Build history of the part. All positions in model axes, mm. A direction names the side the tool comes from. Give positions to 0.01 mm unless a question says otherwise; leave off trailing zeros. Write each loop counter-clockwise with the first axis right and the second up, starting at its lowest first coordinate (ties: lowest second). Pieces come first, ordered by that corner, then holes. Notation, with made-up numbers: (16.5, 11) -> (57.5, 11) arc R11 cw to (57.5, 26) -> close; hole circle Ø3 at (-6, -34.5). An arc over 180 degrees is marked (long way). Put each result on its own line as item: value. Start each with the question number.
Item 1: Flat gauge pins, fed straight in: pin 1 Ø1.4 at (x, z) = (39.5, 1) entering from +Y; pin 2 Ø1 at (x, z) = (-14.5, 2.5) entering from -Y; pin 3 Ø0.8 at (y, z) = (6.5, 1) entering from +X. Where does each tip first touch, or does it go through?
Item 2: Tool access for faces 4 (the flat face through (55.75, -20, 1)), 5 (the flat face through (-17.9, 10, 1)), 6 (the flat face through (0, 26.75, 1)), 7 (the flat face through (29, -26.75, 1)), 8 (the flat face through (17.9, 9, 1)): list every direction of +Z, -Z, +X, -X, +Y, -Y with a clear straight run to the whole face (end or side of a thin tool).
Item 3: Two-plate mould, pull along Y, no slides. Class faces 1 (the cylindrical face through (-4.1, -27.144, 1.38)), 2 (the cylindrical face through (-20.03, -10.26, 0.81)), 3 (the cylindrical face through (24, -12.68, 1.38)): pulls with the +Y half, pulls with the -Y half, needs draft (parallel to the pull), parting line crosses it, or undercut.
Item 4: Drill centre lines: line 1 along X through (y, z) = (-11.25, 1.1); line 2 along X through (y, z) = (-11.25, 2.75); line 3 along Y through (x, z) = (-19.9, 1.05). Where is each one in solid material? Low to high.
Item 5: Slice it at C-C, the plane x = -35. List the corners of the cut face in (y, z), plus the area to 3 significant figures.
Item 6: Slice it at A-A, the plane z = 0.55. List the corners of the cut face in (x, y).
Item 7: Slice it at B-B, the plane y = 3. List the corners of the cut face in (x, z).
```python
from build123d import *

# Parameters (mm, degrees)
BOSS_EXTRUDE1_DEPTH                            = 2.8
CUT_EXTRUDE1_REACH                             = 4.8
SKETCH3_R                                      = 1
CSK_FOR_M2_FLAT_HEAD_MACHINE_SCREW1_AT_2_COUNT = 2
CSK_FOR_M2_FLAT_HEAD_MACHINE_SCREW1_AT_2_PITCH = 39.8


with BuildPart() as part:
    # Sketch1 → Boss-Extrude1 (new body)
    with BuildSketch(Plane.XY):
        with BuildLine():
            Line((-53.75, -26.75), (-5.291502622, -26.75))
            ThreePointArc((-5.291502622, -26.75), (-4.085457244, -27.15455193), (-3.36731985, -28.204545455))
            ThreePointArc((-3.36731985, -28.204545455), (0, -30.75), (3.36731985, -28.204545455))
            ThreePointArc((3.36731985, -28.204545455), (4.085457244, -27.15455193), (5.291502622, -26.75))
            Line((5.291502622, -26.75), (53.75, -26.75))
            ThreePointArc((53.75, -26.75), (55.164213562, -26.164213562), (55.75, -24.75))
            Line((55.75, -24.75), (55.75, -15.25))
            ThreePointArc((55.75, -15.25), (55.164213562, -13.835786438), (53.75, -13.25))
            Line((53.75, -13.25), (25.4, -13.25))
            ThreePointArc((25.4, -13.25), (23.985786438, -12.664213562), (23.4, -11.25))
            ThreePointArc((23.4, -11.25), (22.374873734, -8.775126266), (19.9, -7.75))
            ThreePointArc((19.9, -7.75), (18.485786438, -7.164213562), (17.9, -5.75))
            Line((17.9, -5.75), (17.9, 24.75))
            ThreePointArc((17.9, 24.75), (17.314213562, 26.164213562), (15.9, 26.75))
            Line((15.9, 26.75), (-15.9, 26.75))
            ThreePointArc((-15.9, 26.75), (-17.314213562, 26.164213562), (-17.9, 24.75))
            Line((-17.9, 24.75), (-17.9, -5.75))
            ThreePointArc((-17.9, -5.75), (-18.485786438, -7.164213562), (-19.9, -7.75))
            ThreePointArc((-19.9, -7.75), (-22.374873734, -8.775126266), (-23.4, -11.25))
            ThreePointArc((-23.4, -11.25), (-23.985786438, -12.664213562), (-25.4, -13.25))
            Line((-25.4, -13.25), (-53.75, -13.25))
            ThreePointArc((-53.75, -13.25), (-55.164213562, -13.835786438), (-55.75, -15.25))
            Line((-55.75, -15.25), (-55.75, -24.75))
            ThreePointArc((-55.75, -24.75), (-55.164213562, -26.164213562), (-53.75, -26.75))
        make_face()
    extrude(amount=BOSS_EXTRUDE1_DEPTH)

    # Sketch3 → Cut-Extrude1 (cut, up to next)
    with BuildSketch(Plane.XY.offset(2.8), mode=Mode.PRIVATE) as cut_extrude1_sk1:
        with Locations((-19.9, -11.25)):
            Circle(SKETCH3_R)
    cut_extrude1_tool1 = extrude(cut_extrude1_sk1.sketch, amount=-CUT_EXTRUDE1_REACH, mode=Mode.PRIVATE) & part.part
    add(cut_extrude1_tool1.solids().sort_by_distance((-19.9, -11.25, 2.8))[0], mode=Mode.SUBTRACT)
    # Sketch3 → Cut-Extrude1 (cut, up to next)
    with BuildSketch(Plane.XY.offset(2.8), mode=Mode.PRIVATE) as cut_extrude1_sk2:
        with Locations((19.9, -11.25)):
            Circle(SKETCH3_R)
    cut_extrude1_tool2 = extrude(cut_extrude1_sk2.sketch, amount=-CUT_EXTRUDE1_REACH, mode=Mode.PRIVATE) & part.part
    add(cut_extrude1_tool2.solids().sort_by_distance((19.9, -11.25, 2.8))[0], mode=Mode.SUBTRACT)

    # Sketch4 → CSK for M2 Flat Head Machine Screw1 (revolve, cut)
    with BuildSketch(Plane(origin=(-19.9, -11.25, 2.8), x_dir=(0, -1, 0), z_dir=(1, 0, 0))):
        Polygon((0, 0), (0, 2.8), (1, 2.8), (1, 1.2), (2, 0.2), (2, 0), align=None)
    csk_for_m2_flat_head_machine_screw1 = revolve(axis=Axis((-19.9, -11.25, 9.15), (0, 0, -1)), mode=Mode.SUBTRACT)

    # CSK for M2 Flat Head Machine Screw1 at 2: CSK for M2 Flat Head Machine Screw1 ×2
    with Locations(*[(i * CSK_FOR_M2_FLAT_HEAD_MACHINE_SCREW1_AT_2_PITCH, 0, 0) for i in range(1, CSK_FOR_M2_FLAT_HEAD_MACHINE_SCREW1_AT_2_COUNT)]):
        add(csk_for_m2_flat_head_machine_screw1, mode=Mode.SUBTRACT)


solid = part.part
```
Values follow:
1. pin 1: y = -13.25
1. pin 2: y = -26.75
1. pin 3: x = 17.9
2. face 4: +Z, -Z, +X, +Y, -Y
2. face 5: +Z, -Z, -X, +Y
2. face 6: +Z, -Z, +X, -X, +Y
2. face 7: +Z, -Z, +X, -Y
2. face 8: +Z, -Z, +X, +Y
3. face 1: pulls with the -Y half
3. face 2: undercut
3. face 3: pulls with the +Y half
4. line 1: -23.4 to -20.9, -18.9 to 18.9, 20.9 to 23.4
4. line 2: -23.4 to -21.9, -17.9 to 17.9, 21.9 to 23.4
4. line 3: -26.75 to -12.25, -10.25 to -7.75
5. outline: (-26.75, 0) -> (-13.25, 0) -> (-13.25, 2.8) -> (-26.75, 2.8) -> close
5. area: 37.8 mm2
6. outline: (-55.75, -24.75) arc R2 ccw to (-53.75, -26.75) -> (-5.29, -26.75) arc R2 cw to (-3.37, -28.2) arc R3.5 ccw to (3.37, -28.2) arc R2 cw to (5.29, -26.75) -> (53.75, -26.75) arc R2 ccw to (55.75, -24.75) -> (55.75, -15.25) arc R2 ccw to (53.75, -13.25) -> (25.4, -13.25) arc R2 cw to (23.4, -11.25) arc R3.5 ccw to (19.9, -7.75) arc R2 cw to (17.9, -5.75) -> (17.9, 24.75) arc R2 ccw to (15.9, 26.75) -> (-15.9, 26.75) arc R2 ccw to (-17.9, 24.75) -> (-17.9, -5.75) arc R2 cw to (-19.9, -7.75) arc R3.5 ccw to (-23.4, -11.25) arc R2 cw to (-25.4, -13.25) -> (-53.75, -13.25) arc R2 ccw to (-55.75, -15.25) -> close; hole circle Ø2 at (-19.9, -11.25); hole circle Ø2 at (19.9, -11.25)
7. outline: (-17.9, 0) -> (17.9, 0) -> (17.9, 2.8) -> (-17.9, 2.8) -> close
